Part model, mm, in its own coordinate system. Face numbers are marked on the shaded views. Give positions to 0.01 mm unless a question says otherwise; leave off trailing zeros. Write each loop counter-clockwise with the first axis right and the second up, starting at its lowest first coordinate (ties: lowest second). Pieces come first, ordered by that corner, then holes. Notation, with made-up numbers: (58, 78.25) - (89, 78.25) arc R25 ccw to (89, 98.25) - close; hole circle Ø10 at (37.5, 24.5). An arc over 180 degrees is marked (long way). Answer in a Markdown table with one row per item. Add a question column.
1. Probe line 1 along X through (y, z) = (-6, 1.45); line 2 along X through (y, z) = (-3, 0.9); line 3 along Y through (x, z) = (14.5, 3.5). List the from-to ranges inside material, lowest first.
2. Band-saw the part on A-A on z = 4.25. Write the cut outline in (x, y), plus the area to 3 significant figures.
3. Band-saw the part on B-B on x = 0. State how many separate pieces and enclosed holes the cut face has, plus the area to 3 significant figures.
4. Drop flat-ended pins along their axis: pin 1 Ø2.5 at (x, y) = (0, 9) entering from +Z; pin 2 Ø1.5 at (y, z) = (9.5, 4.5) entering from +X; pin 3 Ø4 at (y, z) = (4, 2.5) entering from +X. Give the stop position or say it passes through.
5. Pull direction Y, two halves, no side cores. Call the marked faces 1, 2 and 3: released by +Y, released by -Y, zero draft, split by the parting line, or undercut.
```python
from build123d import *

# Parameters (mm, degrees)
SKETCH2_R                      = 20.5
BOSS_EXTRUDE1_DEPTH            = 3
SKETCH3_R                      = 18.5
BOSS_EXTRUDE2_DEPTH            = 5
SKETCH4_R                      = 16.5
CUT_EXTRUDE1_DEPTH             = 5
FILLET1_R                      = 1
FILLET2_R                      = 1
SKETCH9_R                      = 1
CUT_EXTRUDE2_DEPTH             = 3
F_2_0MM_DOWEL_HOLE4_AT_2_COUNT = 2
F_2_0MM_DOWEL_HOLE4_AT_2_PITCH = 3
F_2_0MM_DOWEL_HOLE4_AT_3_COUNT = 2
F_2_0MM_DOWEL_HOLE4_AT_3_PITCH = 6
F_2_0MM_DOWEL_HOLE4_AT_4_COUNT = 2
F_2_0MM_DOWEL_HOLE4_AT_4_PITCH = 9
F_2_0MM_DOWEL_HOLE4_AT_5_COUNT = 2
F_2_0MM_DOWEL_HOLE4_AT_5_PITCH = 12
CIRPATTERN1_COUNT              = 6


with BuildPart() as part:
    # Sketch2 → Boss-Extrude1 (new body)
    with BuildSketch(Plane.XY):
        Circle(SKETCH2_R)
    extrude(amount=BOSS_EXTRUDE1_DEPTH)

    # Sketch3 → Boss-Extrude2 (add)
    with BuildSketch(Plane.XY.offset(3)):
        Circle(SKETCH3_R)
    extrude(amount=BOSS_EXTRUDE2_DEPTH)

    # Sketch4 → Cut-Extrude1 (cut)
    with BuildSketch(Plane.XY.offset(8)):
        Circle(SKETCH4_R)
    extrude(amount=-CUT_EXTRUDE1_DEPTH, mode=Mode.SUBTRACT)

    # Fillet1
    fillet1_edges = [part.edges().sort_by_distance(p)[0] for p in [
        (-18.5, 0, 8),
    ]]
    fillet(fillet1_edges, radius=FILLET1_R)

    # Fillet2
    fillet2_edges = [part.edges().sort_by_distance(p)[0] for p in [
        (-20.5, 0, 0),
    ]]
    fillet(fillet2_edges, radius=FILLET2_R)

    # Sketch9 → Cut-Extrude2 (cut)
    with BuildSketch(Plane(origin=(0, 0, 0), x_dir=(-1, 0, 0), z_dir=(0, 0, -1))):
        Circle(SKETCH9_R)
    extrude(amount=-CUT_EXTRUDE2_DEPTH, mode=Mode.SUBTRACT)

    # Sketch12 → Ø2.0mm Dowel Hole4 (revolve, cut)
    with BuildSketch(Plane(origin=(0, 3, 0), x_dir=(0, 1, 0), z_dir=(1, 0, 0))):
        Polygon((0, 0), (0, 100.600860619), (1, 100), (1, 0), align=None)
    f_2_0mm_dowel_hole4 = revolve(axis=Axis((0, 3, -6.35), (0, 0, 1)), mode=Mode.SUBTRACT)

    # Ø2.0mm Dowel Hole4 at 2: Ø2.0mm Dowel Hole4 ×2
    with Locations(*[(0, i * F_2_0MM_DOWEL_HOLE4_AT_2_PITCH, 0) for i in range(1, F_2_0MM_DOWEL_HOLE4_AT_2_COUNT)]):
        add(f_2_0mm_dowel_hole4, mode=Mode.SUBTRACT)

    # Ø2.0mm Dowel Hole4 at 3: Ø2.0mm Dowel Hole4 ×2
    with Locations(*[(0, i * F_2_0MM_DOWEL_HOLE4_AT_3_PITCH, 0) for i in range(1, F_2_0MM_DOWEL_HOLE4_AT_3_COUNT)]):
        add(f_2_0mm_dowel_hole4, mode=Mode.SUBTRACT)

    # Ø2.0mm Dowel Hole4 at 4: Ø2.0mm Dowel Hole4 ×2
    with Locations(*[(0, i * F_2_0MM_DOWEL_HOLE4_AT_4_PITCH, 0) for i in range(1, F_2_0MM_DOWEL_HOLE4_AT_4_COUNT)]):
        add(f_2_0mm_dowel_hole4, mode=Mode.SUBTRACT)

    # Ø2.0mm Dowel Hole4 at 5: Ø2.0mm Dowel Hole4 ×2
    with Locations(*[(0, i * F_2_0MM_DOWEL_HOLE4_AT_5_PITCH, 0) for i in range(1, F_2_0MM_DOWEL_HOLE4_AT_5_COUNT)]):
        add(f_2_0mm_dowel_hole4, mode=Mode.SUBTRACT)

    # CirPattern1: Ø2.0mm Dowel Hole4 ×6 about axis
    cirpattern1_axis = Axis((0, 0, 0), (0, 0, 1))
    for i in range(1, CIRPATTERN1_COUNT):
        add(f_2_0mm_dowel_hole4.rotate(cirpattern1_axis, i * 360 / CIRPATTERN1_COUNT), mode=Mode.SUBTRACT)

    # CirPattern1 copy 1 sketch → CirPattern1 copy 1 (revolve, cut)
    with BuildSketch(Plane(origin=(-5.196152423, 3, 0), x_dir=(-0.866025404, 0.5, 0), z_dir=(0.5, 0.866025404, 0))):
        Polygon((0, 0), (0, 100.600860619), (1, 100), (1, 0), align=None)
    revolve(axis=Axis((-5.196152423, 3, -6.35), (0, 0, 1)), mode=Mode.SUBTRACT)

    # CirPattern1 copy 2 sketch → CirPattern1 copy 2 (revolve, cut)
    with BuildSketch(Plane(origin=(-5.196152423, -3, 0), x_dir=(-0.866025404, -0.5, 0), z_dir=(-0.5, 0.866025404, 0))):
        Polygon((0, 0), (0, 100.600860619), (1, 100), (1, 0), align=None)
    revolve(axis=Axis((-5.196152423, -3, -6.35), (0, 0, 1)), mode=Mode.SUBTRACT)

    # CirPattern1 copy 3 sketch → CirPattern1 copy 3 (revolve, cut)
    with BuildSketch(Plane(origin=(0, -6, 0), x_dir=(0, -1, 0), z_dir=(-1, 0, 0))):
        Polygon((0, 0), (0, 100.600860619), (1, 100), (1, 0), align=None)
    revolve(axis=Axis((0, -6, -6.35), (0, 0, 1)), mode=Mode.SUBTRACT)

    # CirPattern1 copy 4 sketch → CirPattern1 copy 4 (revolve, cut)
    with BuildSketch(Plane(origin=(5.196152423, -3, 0), x_dir=(0.866025404, -0.5, 0), z_dir=(-0.5, -0.866025404, 0))):
        Polygon((0, 0), (0, 100.600860619), (1, 100), (1, 0), align=None)
    revolve(axis=Axis((5.196152423, -3, -6.35), (0, 0, 1)), mode=Mode.SUBTRACT)

    # CirPattern1 copy 5 sketch → CirPattern1 copy 5 (revolve, cut)
    with BuildSketch(Plane(origin=(5.196152423, 3, 0), x_dir=(0.866025404, 0.5, 0), z_dir=(0.5, -0.866025404, 0))):
        Polygon((0, 0), (0, 100.600860619), (1, 100), (1, 0), align=None)
    revolve(axis=Axis((5.196152423, 3, -6.35), (0, 0, 1)), mode=Mode.SUBTRACT)

    # CirPattern1 copy 6 sketch → CirPattern1 copy 6 (revolve, cut)
    with BuildSketch(Plane(origin=(-7.794228634, 4.5, 0), x_dir=(-0.866025404, 0.5, 0), z_dir=(0.5, 0.866025404, 0))):
        Polygon((0, 0), (0, 100.600860619), (1, 100), (1, 0), align=None)
    revolve(axis=Axis((-7.794228634, 4.5, -6.35), (0, 0, 1)), mode=Mode.SUBTRACT)

    # CirPattern1 copy 7 sketch → CirPattern1 copy 7 (revolve, cut)
    with BuildSketch(Plane(origin=(-7.794228634, -4.5, 0), x_dir=(-0.866025404, -0.5, 0), z_dir=(-0.5, 0.866025404, 0))):
        Polygon((0, 0), (0, 100.600860619), (1, 100), (1, 0), align=None)
    revolve(axis=Axis((-7.794228634, -4.5, -6.35), (0, 0, 1)), mode=Mode.SUBTRACT)

    # CirPattern1 copy 8 sketch → CirPattern1 copy 8 (revolve, cut)
    with BuildSketch(Plane(origin=(0, -9, 0), x_dir=(0, -1, 0), z_dir=(-1, 0, 0))):
        Polygon((0, 0), (0, 100.600860619), (1, 100), (1, 0), align=None)
    revolve(axis=Axis((0, -9, -6.35), (0, 0, 1)), mode=Mode.SUBTRACT)

    # CirPattern1 copy 9 sketch → CirPattern1 copy 9 (revolve, cut)
    with BuildSketch(Plane(origin=(7.794228634, -4.5, 0), x_dir=(0.866025404, -0.5, 0), z_dir=(-0.5, -0.866025404, 0))):
        Polygon((0, 0), (0, 100.600860619), (1, 100), (1, 0), align=None)
    revolve(axis=Axis((7.794228634, -4.5, -6.35), (0, 0, 1)), mode=Mode.SUBTRACT)

    # CirPattern1 copy 10 sketch → CirPattern1 copy 10 (revolve, cut)
    with BuildSketch(Plane(origin=(7.794228634, 4.5, 0), x_dir=(0.866025404, 0.5, 0), z_dir=(0.5, -0.866025404, 0))):
        Polygon((0, 0), (0, 100.600860619), (1, 100), (1, 0), align=None)
    revolve(axis=Axis((7.794228634, 4.5, -6.35), (0, 0, 1)), mode=Mode.SUBTRACT)

    # CirPattern1 copy 11 sketch → CirPattern1 copy 11 (revolve, cut)
    with BuildSketch(Plane(origin=(-10.392304845, 6, 0), x_dir=(-0.866025404, 0.5, 0), z_dir=(0.5, 0.866025404, 0))):
        Polygon((0, 0), (0, 100.600860619), (1, 100), (1, 0), align=None)
    revolve(axis=Axis((-10.392304845, 6, -6.35), (0, 0, 1)), mode=Mode.SUBTRACT)

    # CirPattern1 copy 12 sketch → CirPattern1 copy 12 (revolve, cut)
    with BuildSketch(Plane(origin=(-10.392304845, -6, 0), x_dir=(-0.866025404, -0.5, 0), z_dir=(-0.5, 0.866025404, 0))):
        Polygon((0, 0), (0, 100.600860619), (1, 100), (1, 0), align=None)
    revolve(axis=Axis((-10.392304845, -6, -6.35), (0, 0, 1)), mode=Mode.SUBTRACT)

    # CirPattern1 copy 13 sketch → CirPattern1 copy 13 (revolve, cut)
    with BuildSketch(Plane(origin=(0, -12, 0), x_dir=(0, -1, 0), z_dir=(-1, 0, 0))):
        Polygon((0, 0), (0, 100.600860619), (1, 100), (1, 0), align=None)
    revolve(axis=Axis((0, -12, -6.35), (0, 0, 1)), mode=Mode.SUBTRACT)

    # CirPattern1 copy 14 sketch → CirPattern1 copy 14 (revolve, cut)
    with BuildSketch(Plane(origin=(10.392304845, -6, 0), x_dir=(0.866025404, -0.5, 0), z_dir=(-0.5, -0.866025404, 0))):
        Polygon((0, 0), (0, 100.600860619), (1, 100), (1, 0), align=None)
    revolve(axis=Axis((10.392304845, -6, -6.35), (0, 0, 1)), mode=Mode.SUBTRACT)

    # CirPattern1 copy 15 sketch → CirPattern1 copy 15 (revolve, cut)
    with BuildSketch(Plane(origin=(10.392304845, 6, 0), x_dir=(0.866025404, 0.5, 0), z_dir=(0.5, -0.866025404, 0))):
        Polygon((0, 0), (0, 100.600860619), (1, 100), (1, 0), align=None)
    revolve(axis=Axis((10.392304845, 6, -6.35), (0, 0, 1)), mode=Mode.SUBTRACT)

    # CirPattern1 copy 16 sketch → CirPattern1 copy 16 (revolve, cut)
    with BuildSketch(Plane(origin=(-12.990381057, 7.5, 0), x_dir=(-0.866025404, 0.5, 0), z_dir=(0.5, 0.866025404, 0))):
        Polygon((0, 0), (0, 100.600860619), (1, 100), (1, 0), align=None)
    revolve(axis=Axis((-12.990381057, 7.5, -6.35), (0, 0, 1)), mode=Mode.SUBTRACT)

    # CirPattern1 copy 17 sketch → CirPattern1 copy 17 (revolve, cut)
    with BuildSketch(Plane(origin=(-12.990381057, -7.5, 0), x_dir=(-0.866025404, -0.5, 0), z_dir=(-0.5, 0.866025404, 0))):
        Polygon((0, 0), (0, 100.600860619), (1, 100), (1, 0), align=None)
    revolve(axis=Axis((-12.990381057, -7.5, -6.35), (0, 0, 1)), mode=Mode.SUBTRACT)

    # CirPattern1 copy 18 sketch → CirPattern1 copy 18 (revolve, cut)
    with BuildSketch(Plane(origin=(0, -15, 0), x_dir=(0, -1, 0), z_dir=(-1, 0, 0))):
        Polygon((0, 0), (0, 100.600860619), (1, 100), (1, 0), align=None)
    revolve(axis=Axis((0, -15, -6.35), (0, 0, 1)), mode=Mode.SUBTRACT)

    # CirPattern1 copy 19 sketch → CirPattern1 copy 19 (revolve, cut)
    with BuildSketch(Plane(origin=(12.990381057, -7.5, 0), x_dir=(0.866025404, -0.5, 0), z_dir=(-0.5, -0.866025404, 0))):
        Polygon((0, 0), (0, 100.600860619), (1, 100), (1, 0), align=None)
    revolve(axis=Axis((12.990381057, -7.5, -6.35), (0, 0, 1)), mode=Mode.SUBTRACT)

    # CirPattern1 copy 20 sketch → CirPattern1 copy 20 (revolve, cut)
    with BuildSketch(Plane(origin=(12.990381057, 7.5, 0), x_dir=(0.866025404, 0.5, 0), z_dir=(0.5, -0.866025404, 0))):
        Polygon((0, 0), (0, 100.600860619), (1, 100), (1, 0), align=None)
    revolve(axis=Axis((12.990381057, 7.5, -6.35), (0, 0, 1)), mode=Mode.SUBTRACT)


solid = part.part
```
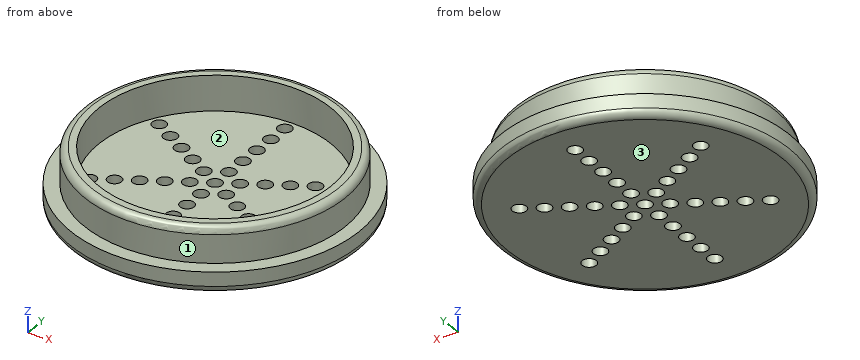
Values:
| question | item | result |
|---|---|---|
| 1 | line 1 | x = -19.6 to -11.39, -9.39 to -1, 1 to 9.39, 11.39 to 19.6 |
| 1 | line 2 | x = -20.27 to -6.2, -4.2 to -1, 1 to 4.2, 6.2 to 20.27 |
| 1 | line 3 | y = -11.49 to -7.87, 7.87 to 11.49 |
| 2 | outline | circle Ø37 at (0, 0); hole circle Ø33 at (0, 0) |
| 2 | area | 220 mm² |
| 3 | separate pieces | 12 |
| 3 | enclosed holes | 0 |
| 3 | area | 76.1 mm² |
| 4 | pin 1 | stops at z = 3 |
| 4 | pin 2 | stops at x = 16.3 |
| 4 | pin 3 | stops at x = 20.4 |
| 5 | face 1 | split by the parting line |
| 5 | face 2 | undercut |
| 5 | face 3 | zero draft |
